from build123d import *

# Parameters (mm, degrees)
BASE_FLANGE1_DEPTH         = 38.1
F_6_0_204_DIAMETER_HOLE1_D = 5.1816
F_6_0_204_DIAMETER_HOLE2_D = 5.1816


# Sheet-metal steps are written as plain solids
with BuildPart() as part:
    # Sketch1 → Base-Flange1 (new body)
    with BuildSketch(Plane(origin=(0, 0, 0), x_dir=(1, 0, 0), z_dir=(0, 1, 0))):
        with BuildLine():
            Line((0, 0), (-19.667225995, 0))
            ThreePointArc((-19.667225995, 0), (-19.992101306, 0.035603868), (-20.301554193, 0.14072529))
            Line((-20.301554193, 0.14072529), (-49.839171097, 13.924946512))
            ThreePointArc((-49.839171097, 13.924946512), (-50.004212637, 13.981011271), (-50.177479469, 14))
            Line((-50.177479469, 14), (-70, 14))
            Line((-70, 14), (-70, 14.7))
            Line((-70, 14.7), (-50.177479469, 14.7))
            ThreePointArc((-50.177479469, 14.7), (-49.852604159, 14.664396132), (-49.543151271, 14.55927471))
            Line((-49.543151271, 14.55927471), (-20.005534367, 0.775053488))
            ThreePointArc((-20.005534367, 0.775053488), (-19.840492827, 0.718988729), (-19.667225995, 0.7))
            Line((-19.667225995, 0.7), (0, 0.7))
            Line((0, 0.7), (0, 0))
        make_face()
    extrude(amount=BASE_FLANGE1_DEPTH)

    # #6 (0.204) Diameter Hole1 (through all)
    with Locations(Plane(origin=(0, 0, -0.7), x_dir=(-1, 0, 0), z_dir=(0, 0, -1))):
        with Locations((10, 29.05), (10, 19.05), (10, 9.05)):
            Hole(F_6_0_204_DIAMETER_HOLE1_D / 2)

    # #6 (0.204) Diameter Hole2 (through all)
    with Locations(Plane(origin=(0, 0, -14.7), x_dir=(-1, 0, 0), z_dir=(0, 0, -1))):
        with Locations((59.259333943, 26.55), (59.936433657, 11.55)):
            Hole(F_6_0_204_DIAMETER_HOLE2_D / 2)


solid = part.part
Could you check a few things on this model? Use its own coordinates, in mm. A direction names the side the tool comes from. Give positions to 0.01 mm unless a question says otherwise; leave off trailing zeros. Order: outer loops, then holes, each group sorted by start corner. A loop starts at its lowest first (then second) coordinate and runs counter-clockwise, first axis right, second up.
1. Will these pins go through, and if not, where does the flat tip stop? P1, Ø8.5, axis at x = -10, y = 19.05, coming from the -Z side; P2, Ø2, axis at y = 17.5, z = -2, coming from the -X side; P3, Ø6, axis at x = -28, y = 21.5, coming from the +Z side; P4, Ø4, axis at x = -59.94, y = 11.55, coming from the +Z side (1 decimal).
2. Suppose I cut it at A-A (x = -10). List the corners of the cut face in (y, z) for me.
3. Suppose I cut it at C-C (z = -12.5). List the corners of the cut face in (x, y) for me.
4. For faces 1 (the flat face through (-34.8, 0, -7.4)), 2 (the flat face through (-10, 23, -0.7)), which set-ups out of +Z, -Z, +X, -X, +Y, -Y let a thin tool reach every point of the face, with its end or its side?
5. We'd pull the mould along X, two halves only. Please class faces 3 (the cylindrical face through (-61.17, 28.3, -14.35)), 4 (the cylindrical face through (-57.543, 10.558, -14.345)), 5 (the flat face through (-35, 19, -7)), 6 (the flat face through (-60, 19, -14)): pulls with the +X half, pulls with the -X half, needs draft (parallel to the pull), parting line crosses it, or undercut.
6. Suppose I cut it at B-B (y = 19.05). List the corners of the cut face in (x, z) for me.
7. Suppose I cut it at D-D (x = -45.5). List the corners of the cut face in (y, z) for me, plus the area to 3 significant figures.
8. I need wall thicknesses on L1, parallel to Y at x = -10, z = -0.4; L2, parallel to Z at x = -15, y = 30.5; L3, parallel to Z at x = -65, y = 7. Which ranges of each line are inside material? Lowest first, please.
Solved:
1. P1: stops at z = -0.7
1. P2: stops at x = -26.43
1. P3: stops at z = -2.33
1. P4: passes through
2. outline: (0, -0.7) - (6.46, -0.7) - (6.46, 0) - (0, 0) - close; (11.64, -0.7) - (16.46, -0.7) - (16.46, 0) - (11.64, 0) - close; (21.64, -0.7) - (26.46, -0.7) - (26.46, 0) - (21.64, 0) - close; (31.64, -0.7) - (38.1, -0.7) - (38.1, 0) - (31.64, 0) - close
3. outline: (-46.79, 0) - (-45.13, 0) - (-45.13, 38.1) - (-46.79, 38.1) - close
4. face 1: +Z, -Z, +X, -X, -Y
4. face 2: -Z, +X, +Y, -Y
5. face 3: undercut
5. face 4: undercut
5. face 5: pulls with the -X half
5. face 6: needs draft
6. outline: (-70, -14.7) - (-50.18, -14.7) arc R1.5 ccw to (-49.54, -14.56) - (-20.01, -0.78) arc R0.8 cw to (-19.67, -0.7) - (-12.59, -0.7) - (-12.59, 0) - (-19.67, 0) arc R1.5 ccw to (-20.3, -0.14) - (-49.84, -13.92) arc R0.8 cw to (-50.18, -14) - (-70, -14) - close; (-7.41, -0.7) - (0, -0.7) - (0, 0) - (-7.41, 0) - close
7. outline: (0, -12.67) - (38.1, -12.67) - (38.1, -11.9) - (0, -11.9) - close
7. area: 29.4 mm2
8. L1: y = 0 to 6.46, 11.64 to 16.46, 21.64 to 26.46, 31.64 to 38.1
8. L2: z = -0.7 to 0
8. L3: z = -14.7 to -14
